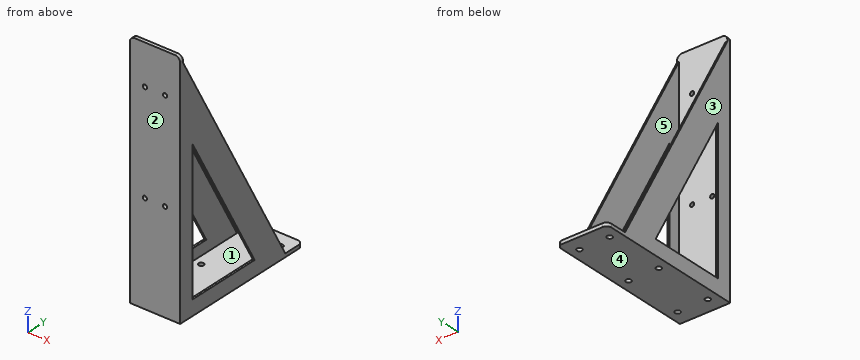
```python
from build123d import *

# Parameters (mm, degrees)
EXTRUDE_1_DEPTH     = 25
SKETCH_4_R          = 2.6
CUT_EXTRUDE_2_DEPTH = 241
FILLET_1_R          = 5
FILLET_2_R          = 5
SKETCH_5_R          = 2.1
CUT_EXTRUDE_3_DEPTH = 151
EXTRUDE_2_DEPTH     = 2
EXTRUDE_3_DEPTH     = 2
CUT_EXTRUDE_4_DEPTH = 51


with BuildPart() as part:
    # 草图1 → 凸台-拉伸1 (new body, symmetric)
    with BuildSketch(Plane(origin=(0, 0, 0), x_dir=(0, 0, -1), z_dir=(1, 0, 0))):
        Polygon((-240, 0), (0, 0), (0, 150), (-3.5, 150), (-3.5, 3.5), (-240, 3.5), align=None)
    extrude(amount=EXTRUDE_1_DEPTH, both=True)

    # 草图4 → 切除-拉伸2 (cut, through all)
    with BuildSketch(Plane(origin=(0, 0, 0), x_dir=(-1, 0, 0), z_dir=(0, 0, -1))):
        with Locations((-15, 135)):
            Circle(SKETCH_4_R)
        with Locations((15, 135)):
            Circle(SKETCH_4_R)
        with Locations((15, 15)):
            Circle(SKETCH_4_R)
        with Locations((-15, 15)):
            Circle(SKETCH_4_R)
        with Locations((-15, 75)):
            Circle(SKETCH_4_R)
        with Locations((15, 75)):
            Circle(SKETCH_4_R)
    extrude(amount=-CUT_EXTRUDE_2_DEPTH, mode=Mode.SUBTRACT)

    # 圆角1
    fillet_1_edges = [part.edges().sort_by_distance(p)[0] for p in [
        (25, 1.75, 240),
        (-25, 1.75, 240),
    ]]
    fillet(fillet_1_edges, radius=FILLET_1_R)

    # 圆角2
    fillet_2_edges = [part.edges().sort_by_distance(p)[0] for p in [
        (25, 150, 1.75),
        (-25, 150, 1.75),
    ]]
    fillet(fillet_2_edges, radius=FILLET_2_R)

    # 草图5 → 切除-拉伸3 (cut, through all)
    with BuildSketch(Plane.XZ):
        with Locations((-10, 200)):
            Circle(SKETCH_5_R)
        with Locations((-10, 100)):
            Circle(SKETCH_5_R)
        with Locations((10, 100)):
            Circle(SKETCH_5_R)
        with Locations((10, 200)):
            Circle(SKETCH_5_R)
    extrude(amount=-CUT_EXTRUDE_3_DEPTH, mode=Mode.SUBTRACT)

    # 草图8 → 凸台-拉伸2 (add)
    with BuildSketch(Plane(origin=(25, 0, 0), x_dir=(0, 0, -1), z_dir=(1, 0, 0))):
        Polygon((-3.5, 3.5), (-233.5, 3.5), (-3.5, 128.5), align=None)
    extrude(amount=-EXTRUDE_2_DEPTH)

    # 草图9 → 凸台-拉伸3 (add)
    with BuildSketch(Plane.ZY.offset(25)):
        Polygon((3.5, 3.5), (233.5, 3.5), (3.5, 128.5), align=None)
    extrude(amount=-EXTRUDE_3_DEPTH)

    # 草图10 → 切除-拉伸4 (cut, through all)
    with BuildSketch(Plane.ZY.offset(25)):
        Polygon((15, 91.086956522), (15, 15), (155, 15), align=None)
    extrude(amount=-CUT_EXTRUDE_4_DEPTH, mode=Mode.SUBTRACT)


solid = part.part
```
Verification items for the finished model (mm, model axes). Face numbers are marked on the shaded views. A direction names the side the tool comes from. Coordinates: 2 decimals unless noted, no trailing zeros. Loops run counter-clockwise (first coordinate to the right, second up) from the corner with the lowest first, then second, coordinate; pieces in that order, holes last. Notation, with made-up numbers: (67, 74) - (102, 74) arc R17 ccw to (102, 100) - close; hole circle Ø2 at (-15, 59.25). An arc over 180 degrees is marked (long way). Answer as a JSON object with one key per item and string values.
(1) Mould release check, pull along X, two halves, no side actions. Record for the marked faces 1, 2 and 3: pulls with the +X half, pulls with the -X half, needs draft (parallel to the pull), parting line crosses it, or undercut.
Response:
{"face 1": "undercut", "face 2": "needs draft", "face 3": "pulls with the -X half"}
(2) Cross-section at D-D, the plane y = 75. Record the boundary of the cut face in (x, z), then the cut area to 3 significant figures.
Response:
{"outline": "(-25, 0) - (-17.6, 0) - (-17.6, 3.5) - (-23, 3.5) - (-23, 15) - (-25, 15) - close; (-25, 44.6) - (-23, 44.6) - (-23, 101.94) - (-25, 101.94) - close; (-12.4, 0) - (12.4, 0) - (12.4, 3.5) - (-12.4, 3.5) - close; (17.6, 0) - (25, 0) - (25, 15) - (23, 15) - (23, 3.5) - (17.6, 3.5) - close; (23, 44.6) - (25, 44.6) - (25, 101.94) - (23, 101.94) - close", "area": "414 mm²"}
(3) Scan lines: line 1 along X through (y, z) = (135, 1.5); line 2 along Y through (x, z) = (-15, 2.6); line 3 along Z through (x, y) = (10, 2.8). Record each from-to range of solid material in increasing order.
Response:
{"line 1": "x = -25 to -17.6, -12.4 to 12.4, 17.6 to 25", "line 2": "y = 0 to 12.4, 17.6 to 72.4, 77.6 to 132.4, 137.6 to 150", "line 3": "z = 0 to 97.9, 102.1 to 197.9, 202.1 to 240"}
(4) Access from +Z, -Z, +X, -X, +Y, -Y to the whole of each face (thin tool, end or side, straight path). Record for the marked faces 4 and 5.
Response:
{"face 4": "-Z, +X, -X, +Y, -Y", "face 5": "+Z, +Y"}
(5) Cross-section at B-B, the plane x = -15. Record the boundary of the cut face in (y, z).
Response:
{"outline": "(0, 0) - (12.4, 0) - (12.4, 3.5) - (3.5, 3.5) - (3.5, 240) - (0, 240) - close; (17.6, 0) - (72.4, 0) - (72.4, 3.5) - (17.6, 3.5) - close; (77.6, 0) - (132.4, 0) - (132.4, 3.5) - (77.6, 3.5) - close; (137.6, 0) - (150, 0) - (150, 3.5) - (137.6, 3.5) - close"}
(6) Cross-section at C-C, the plane z = 222. Record the boundary of the cut face in (x, y).
Response:
{"outline": "(-25, 0) - (25, 0) - (25, 9.75) - (23, 9.75) - (23, 3.5) - (-23, 3.5) - (-23, 9.75) - (-25, 9.75) - close"}
(7) Go/stop test with flat-tipped pins: pin 1 Ø1 at (x, z) = (24, 77) entering from +Y; pin 2 Ø1.6 at (x, y) = (24, 64.5) entering from +Z; pin 3 Ø6 at (x, y) = (-15, 135) entering from +Z; pin 4 Ø4.5 at (x, y) = (15, 75) entering from +Z. Record where each tip stops, or that it passes through.
Response:
{"pin 1": "stops at y = 88.83", "pin 2": "stops at z = 122.73", "pin 3": "stops at z = 3.5", "pin 4": "passes through"}
(8) Cross-section at A-A, the plane y = 135. Record the boundary of the cut face in (x, z), then the cut area to 3 significant figures.
Response:
{"outline": "(-25, 0) - (-17.6, 0) - (-17.6, 3.5) - (-25, 3.5) - close; (-12.4, 0) - (12.4, 0) - (12.4, 3.5) - (-12.4, 3.5) - close; (17.6, 0) - (25, 0) - (25, 3.5) - (17.6, 3.5) - close", "area": "139 mm²"}
